Read the model definition and answer for the solid it produces. Units are mm, in the model's axes. Face numbers are marked on the shaded views. A direction names the side the tool comes from. Round coordinates to 2 decimals unless told otherwise and drop trailing zeros. Order: outer loops, then holes, each group sorted by start corner. A loop starts at its lowest first (then second) coordinate and runs counter-clockwise, first axis right, second up. Notation, with made-up numbers: (67.5, -1.5) -> (117.5, -1.5) arc R19 cw to (117.5, 6.5) -> close; hole circle Ø11 at (-10.5, -35). An arc over 180 degrees is marked (long way). Answer as a JSON object with one key per item and string values. Group by question number.
Item 1: Section C-C, the plane y = -5 is taken. Write down the section's boundary in (x, z), plus the area to 3 significant figures.
Item 2: Section B-B, the plane z = -4.5 is taken. Write down the section's boundary in (x, y), plus the area to 3 significant figures.
Item 3: Section D-D, the plane x = -8.5 is taken. Write down the section's boundary in (y, z).
Item 4: The mould has two halves that part along Z. Classify the marked faces 3, 4 and 5: pulls with the +Z half, pulls with the -Z half, needs draft (parallel to the pull), parting line crosses it, or undercut.
Item 5: For the marked faces 1 and 2, determine the directions among +Z, -Z, +X, -X, +Y, -Y from which every point of the face is accessible in a straight line to the end or side of a thin tool.
Item 6: Section A-A, the plane z = 0 is taken. Write down the section's boundary in (x, y), plus the area to 3 significant figures.
Item 7: Consider probe 1 along Y at (x, z) = (-17, 0.5); probe 2 along X at (y, z) = (-8.5, 5); probe 3 along X at (y, z) = (13.75, 0). Determine where each line is inside the solid, lowest interval first. Write a range as from..to.
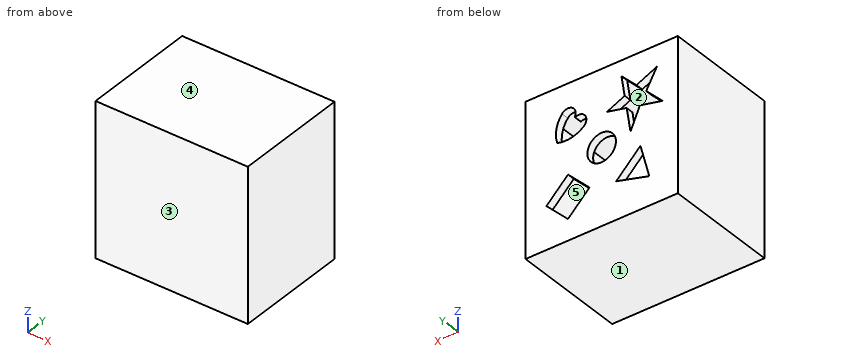
from build123d import *

# Parameters (mm, degrees)
SKETCH1_W           = 40
SKETCH1_H           = 40
BOSS_EXTRUDE1_DEPTH = 15
SKETCH2_W           = 36
SKETCH2_H           = 36
CUT_EXTRUDE1_DEPTH  = 26
SKETCH4_R           = 3.75
CUT_EXTRUDE4_DEPTH  = 2
FILLET1_R           = 0.1


with BuildPart() as part:
    # Sketch1 → Boss-Extrude1 (new, symmetric)
    with BuildSketch(Plane(origin=(0, 0, 0), x_dir=(1, 0, 0), z_dir=(0, 1, 0))):
        Rectangle(SKETCH1_W, SKETCH1_H)
    extrude(amount=BOSS_EXTRUDE1_DEPTH, both=True)

    # Sketch2 → Cut-Extrude1 (cut)
    with BuildSketch(Plane(origin=(0, 13, 0), x_dir=(1, 0, 0), z_dir=(0, 1, 0))):
        Rectangle(SKETCH2_W, SKETCH2_H)
    extrude(amount=-CUT_EXTRUDE1_DEPTH, mode=Mode.SUBTRACT)

    # Sketch4 → Cut-Extrude4 (cut)
    with BuildSketch(Plane(origin=(0, 15, 0), x_dir=(1, 0, 0), z_dir=(0, 1, 0))):
        with Locations(Location((0, 0, 0), (0, 0, 270))):
            Circle(SKETCH4_R)
        Polygon((-15.997574875, -5.191274493), (-10.056879788, -6.527978961), (-7.581971152, -0.903310223), (-6.566729947, -7.313290918), (-1.363004172, -8.484171327), (-6.041352713, -10.630392221), (-5.191274493, -15.997574875), (-9.13789809, -12.050951278), (-14.520043083, -14.520043083), (-11.706657929, -9.482191438), align=None)
        Polygon((14.495689014, 8.838834765), (8.838834765, 14.495689014), (3.181980515, 8.838834765), (8.838834765, 3.181980515), align=None)
        Polygon((-12.513069379, 12.513069379), (-10.183697973, 3.819736942), (-3.819736942, 10.183697973), align=None)
        with BuildLine():
            ThreePointArc((10.41110341, -12.903373255), (11.893574864, -9.612592954), (11.66726189, -6.01040764))
            ThreePointArc((11.66726189, -6.01040764), (8.065076576, -5.784094666), (4.774296275, -7.26656612))
            ThreePointArc((4.774296275, -7.26656612), (4.514513562, -10.166351585), (7.424621202, -10.253048327))
            ThreePointArc((7.424621202, -10.253048327), (7.511317945, -13.163155967), (10.41110341, -12.903373255))
        make_face()
    extrude(amount=-CUT_EXTRUDE4_DEPTH, mode=Mode.SUBTRACT)

    # Fillet1
    fillet1_edges = [part.edges().sort_by_distance(p)[0] for p in [
        (7.424621202, 14, 10.253048327),
    ]]
    fillet(fillet1_edges, radius=FILLET1_R)


solid = part.part
Values found:
{
 "1": {"outline": "(-20, -20) -> (20, -20) -> (20, 20) -> (-20, 20) -> close; hole (-18, -18) -> (18, -18) -> (18, 18) -> (-18, 18) -> close", "area": "304 mm2"},
 "2": {"outline": "(-20, -15) -> (20, -15) -> (20, 15) -> (10.16, 15) -> (10.16, 13) -> (18, 13) -> (18, -13) -> (-18, -13) -> (-18, 13) -> (-10.37, 13) -> (-10.37, 15) -> (-20, 15) -> close; (-9.5, 13) -> (7.52, 13) -> (7.52, 15) -> (-9.5, 15) -> close", "area": "257 mm2"},
 "3": {"outline": "(-15, -20) -> (15, -20) -> (15, -11.44) -> (13, -11.44) -> (13, -18) -> (-13, -18) -> (-13, 18) -> (13, 18) -> (13, 12.69) -> (15, 12.69) -> (15, 20) -> (-15, 20) -> close; (13, -5.5) -> (15, -5.5) -> (15, 2.99) -> (13, 2.99) -> close"},
 "4": {"face 3": "needs draft", "face 4": "pulls with the +Z half", "face 5": "undercut"},
 "5": {"face 1": "-Z, +X, -X, +Y, -Y", "face 2": "none"},
 "6": {"outline": "(-20, -15) -> (20, -15) -> (20, 15) -> (3.75, 15) -> (3.75, 13) -> (18, 13) -> (18, -13) -> (-18, -13) -> (-18, 13) -> (-3.75, 13) -> (-3.75, 15) -> (-20, 15) -> close", "area": "249 mm2"},
 "7": {"probe 1": "-15..-13, 13..15", "probe 2": "-20..-18, 18..20", "probe 3": "-20..-3.75, 3.75..20"}
}
